Autodesk Inventor part; units mm, degrees
ref_plane "YZ Plane" through (0, 0, 0) normal (1, 0, 0) x (0, 1, 0)
ref_plane "XZ Plane" through (0, 0, 0) normal (0, 1, 0) x (-1, 0, 0)
ref_plane "XY Plane" through (0, 0, 0) normal (0, 0, 1) x (1, 0, 0)
sketch "Sketch1" plane through (0, 0, 0) normal (0, 0, 1) x (1, 0, 0)
  circle A0 centre (0, 0) radius 38.1
  dimension "d0" = 76.2
extrude "Extrusion1" add sketch "Sketch1" along normal blind 6.35
sketch "Sketch2" plane through (0, 0, 6.35) normal (0, 0, 1) x (1, 0, 0)
  circle A0 centre (0, 0) radius 38.1
  circle A1 centre (0, 31.75) radius 3.175
  dimension "d3" = 6.35
  dimension "d6" = 31.75
extrude "Extrusion2" cut sketch "Sketch2" against normal through all contours A1
sketch "Sketch3" plane through (0, 0, 6.35) normal (0, 0, 1) x (1, 0, 0)
  circle A0 centre (0, 31.75) radius 3.175
  line L0 (0, 31.75) -> (1.27, 31.75)
  line L1 (1.27, 31.75) -> (1.27, 26.67)
  line L2 (1.27, 26.67) -> (0, 26.67)
  line L3 (0, 26.67) -> (0, 31.75)
  line L4 (0, 31.75) -> (-1.27, 31.75)
  line L5 (-1.27, 31.75) -> (-1.27, 26.67)
  line L6 (-1.27, 26.67) -> (0, 26.67)
  line L7 (0, 26.67) -> (0, 31.75)
  dimension "d9" = 1.27
  dimension "d10" = 5.08
extrude "Extrusion3" cut sketch "Sketch3" against normal through all contours L5 L4 L3 A0 | A0 L3 L6 L5 | L1 L2 L3 A0 | A0 L3 L0 L1
properties part number "Circular Pattern"
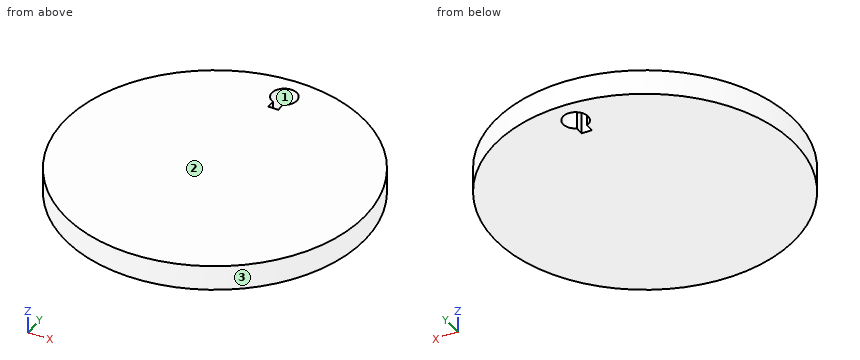
The model under review builds one solid part; all positions refer to its coordinate system, in mm. Face numbers are marked on the shaded views. Round coordinates to 2 decimals unless told otherwise and drop trailing zeros. Write each loop counter-clockwise with the first axis right and the second up, starting at its lowest first coordinate (ties: lowest second). Pieces come first, ordered by that corner, then holes. Notation, with made-up numbers: (8.25, 7) - (31.25, 7) arc R10 cw to (31.25, 18) - close; hole circle Ø9 at (-11.5, -24). An arc over 180 degrees is marked (long way). Answer as CSV lines item,"result". Start each with the question number.
(1) For pin 1 Ø1.3 at (x, z) = (0, 4.5) entering from +Y; pin 2 Ø5 at (x, y) = (15, 13.5) entering from -Z; pin 3 Ø1.7 at (y, z) = (28, 4) entering from +X; pin 4 Ø2 at (y, z) = (-2.5, 3.5) entering from -X, all flat-tipped, find the tip position at first contact; note any pin that passes through.
(2) Draft analysis for pull direction Y (two halves, no side actions). For the marked faces 1, 2 and 3, state which applies: pulls with the +Y half, pulls with the -Y half, needs draft (parallel to the pull), parting line crosses it, or undercut.
(3) To check wall thickness, follow line 1 (Y direction, x = 0, z = 4.5) (3 decimals); line 2 (X direction, y = 32, z = 3.25); line 3 (X direction, y = 27.5, z = 2.25). State the ranges of each line that lie inside material, in increasing order.
(4) We need section A-A on x = 0. State the section outline as (y, z) points (3 decimals), plus the area to 3 significant figures.
(5) We need section D-D on x = 22. State the section outline as (y, z) points.
(6) We need section B-B on z = 1.75. State the section outline as (x, y) points (3 decimals), plus the area to 3 significant figures.
(7) We need section C-C on y = 31.75. State the section outline as (x, z) points (3 decimals), plus the area to 3 significant figures.
Worked answers:
1,pin 1,"y = 38.1"
1,pin 2,"z = 0"
1,pin 3,"x = 26.73"
1,pin 4,"x = -38.07"
2,face 1,"undercut"
2,face 2,"needs draft"
2,face 3,"parting line crosses it"
3,line 1,"-38.1 to 26.67, 34.925 to 38.1"
3,line 2,"-20.68 to -3.17, 3.17 to 20.68"
3,line 3,"-26.37 to -1.27, 1.27 to 26.37"
4,outline,"(-38.1, 0) - (26.67, 0) - (26.67, 6.35) - (-38.1, 6.35) - close; (34.925, 0) - (38.1, 0) - (38.1, 6.35) - (34.925, 6.35) - close"
4,area,"431 mm²"
5,outline,"(-31.11, 0) - (31.11, 0) - (31.11, 6.35) - (-31.11, 6.35) - close"
6,outline,"circle Ø76.2 at (0, 0); hole (-1.27, 26.67) - (1.27, 26.67) - (1.27, 28.84) arc R3.175 ccw (long way) to (-1.27, 28.84) - close"
6,area,"4,520 mm²"
7,outline,"(-21.061, 0) - (-3.175, 0) - (-3.175, 6.35) - (-21.061, 6.35) - close; (3.175, 0) - (21.061, 0) - (21.061, 6.35) - (3.175, 6.35) - close"
7,area,"227 mm²"
